from build123d import *

# Parameters (mm, degrees)
BOSS_EXTRU_1_DEPTH           = 20
ESQUISSE1_4_R                = 14
ENL_V_MAT_EXTRU_1_DEPTH      = 8
ESQUISSE3_R                  = 5
ENL_V_MAT_EXTRU_2_DEPTH      = 14
ENL_V_MAT_EXTRU_3_DEPTH      = 42.231056256
ENL_V_MAT_EXTRU_3_DEPTH_BACK = 42.231056256
ESQUISSE1_5_R                = 2
ESQUISSE1_6_R                = 4
ENL_V_MAT_EXTRU_4_DEPTH      = 2
ENL_V_START                  = 18
ESQUISSE1_7_R                = 4
ENL_V_MAT_EXTRU_5_DEPTH      = 2
ENL_V_MAT_EXTRU_6_REACH      = 43.231
ESQUISSE4_R                  = 10
ENL_V_MAT_EXTRU_7_DEPTH      = 8


with BuildPart() as part:
    # Esquisse1 → Boss.-Extru.1 (new body)
    with BuildSketch(Plane.XY):
        with BuildLine():
            Line((0, 20), (-30, 20))
            Line((-30, 20), (-30, -20))
            Line((-30, -20), (0, -20))
            ThreePointArc((0, -20), (20, 0), (0, 20))
        make_face()
    extrude(amount=BOSS_EXTRU_1_DEPTH)

    # Esquisse1<4> → Enlèv. mat.-Extru.1 (cut)
    with BuildSketch(Plane.XY):
        Circle(ESQUISSE1_4_R)
    extrude(amount=ENL_V_MAT_EXTRU_1_DEPTH, mode=Mode.SUBTRACT)

    # Esquisse3 → Enlèv. mat.-Extru.2 (cut)
    with BuildSketch(Plane.ZY.offset(30)):
        with Locations((10, 0)):
            Circle(ESQUISSE3_R)
    extrude(amount=-ENL_V_MAT_EXTRU_2_DEPTH, mode=Mode.SUBTRACT)

    # Esquisse1<5> → Enlèv. mat.-Extru.3 (cut, two sides: drawn at the far end of the back side and taken through both)
    with BuildSketch(Plane.XY.offset(-ENL_V_MAT_EXTRU_3_DEPTH_BACK)):
        with Locations((-23.5, 0)):
            Circle(ESQUISSE1_5_R)
    extrude(amount=ENL_V_MAT_EXTRU_3_DEPTH + ENL_V_MAT_EXTRU_3_DEPTH_BACK, mode=Mode.SUBTRACT)

    # Esquisse1<6> → Enlèv. mat.-Extru.4 (cut)
    with BuildSketch(Plane.XY):
        with Locations((-23.5, 0)):
            Circle(ESQUISSE1_6_R)
    extrude(amount=ENL_V_MAT_EXTRU_4_DEPTH, mode=Mode.SUBTRACT)

    # Esquisse1<7> → Enlèv. mat.-Extru.5 (cut)
    with BuildSketch(Plane.XY.offset(ENL_V_START)):
        with Locations((-23.5, 0)):
            Circle(ESQUISSE1_7_R)
    extrude(amount=ENL_V_MAT_EXTRU_5_DEPTH, mode=Mode.SUBTRACT)

    # Esquisse4 → Enlèv. mat.-Extru.6 (cut, up to next)
    with BuildSketch(Plane.XY.offset(20), mode=Mode.PRIVATE) as enl_v_mat_extru_6_sk1:
        Circle(ESQUISSE4_R)
    enl_v_mat_extru_6_tool1 = extrude(enl_v_mat_extru_6_sk1.sketch, amount=-ENL_V_MAT_EXTRU_6_REACH, mode=Mode.PRIVATE) & part.part
    add(enl_v_mat_extru_6_tool1.solids().sort_by_distance((0, 0, 20))[0], mode=Mode.SUBTRACT)

    # Esquisse5 → Enlèv. mat.-Extru.7 (cut)
    with BuildSketch(Plane.XY.offset(20)):
        with BuildLine():
            Line((0, 10), (0, 20))
            ThreePointArc((0, 20), (20, 0), (0, -20))
            Line((0, -20), (0, -10))
            ThreePointArc((0, -10), (-10, 0), (0, 10))
        make_face()
    extrude(amount=-ENL_V_MAT_EXTRU_7_DEPTH, mode=Mode.SUBTRACT)


solid = part.part
Check sheet for the modelled part. Datum: model origin and axes. Units: mm. A direction names the side the tool comes from. Give positions to 0.01 mm unless a question says otherwise; leave off trailing zeros. Write each loop counter-clockwise with the first axis right and the second up, starting at its lowest first coordinate (ties: lowest second). Pieces come first, ordered by that corner, then holes. Notation, with made-up numbers: (-3.5, 17) -> (5.5, 17) arc R20 ccw to (5.5, 53) -> close; hole circle Ø6 at (37, -11.75). An arc over 180 degrees is marked (long way). One line per item, written item: value. Start each with the question number.
Item 1: Section check B-B on x = -23.5. Record the cut outline in (y, z), then the cut area to 3 significant figures.
Item 2: Tool access check on faces 1 (the cylindrical face through (-23.098, -4.436, 12.307)), 2 (the cylindrical face through (-26.7, -2.4, 19)), 3 (the flat face through (0, 15, 16)), 4 (the cylindrical face through (12.932, -5.362, 3.944)). Record the directions out of +Z, -Z, +X, -X, +Y, -Y that give a thin tool (end or side, any length) a straight path to the whole face; none if there is none.
Item 3: Gauge pin test, flat ends, axial feed: pin 1 (9 mm diameter, centred on y = 13, z = 17.5, fed in from +X); pin 2 (9 mm diameter, centred on y = -16, z = 14, fed in from +X); pin 3 (18 mm diameter, centred on x = 0, y = 0, fed in from +Z); pin 4 (4 mm diameter, centred on x = -24, y = 1, fed in from -Z). Record the tip position at first contact, or that the pin passes through.
Item 4: Draft check along Y on faces 5 (the flat face through (-15, 0, 20)), 6 (the cylindrical face through (-21.592, 0.601, 3.685)), 7 (the flat face through (-15, 20, 10)). Enter one of: +Y half, -Y half, draft (parallel to the pull), parting line (faces both ways), or undercut.
Item 5: Section check A-A on z = 10. Record the cut outline in (x, y).
Item 6: Section check C-C on y = 0. State how many separate pieces and enclosed holes the cut face has, then the cut area to 3 significant figures.
Item 7: Material ranges on probe 1 along X at (y, z) = (0, 10.65); probe 2 along Y at (x, z) = (-23.5, 17.05); probe 3 along Y at (x, z) = (0, 10.5), recorded low to high. Write a range as from..to.
Item 8: Section check D-D on x = -17.5. Record the cut outline in (y, z), then the cut area to 3 significant figures.
Results list:
1. outline: (-20, 0) -> (-4, 0) -> (-4, 2) -> (-2, 2) -> (-2, 5.42) arc R5 cw to (-2, 14.58) -> (-2, 18) -> (-4, 18) -> (-4, 20) -> (-20, 20) -> close; (2, 2) -> (4, 2) -> (4, 0) -> (20, 0) -> (20, 20) -> (4, 20) -> (4, 18) -> (2, 18) -> (2, 14.58) arc R5 cw to (2, 5.42) -> close
1. area: 664 mm²
2. face 1: -X
2. face 2: +Z
2. face 3: +Z, +X, +Y, -Y
2. face 4: -Z
3. pin 1: x = 0
3. pin 2: x = 16.02
3. pin 3: through
3. pin 4: z = 2
4. face 5: draft
4. face 6: undercut
4. face 7: +Y half
5. outline: (-30, -20) -> (0, -20) arc R20 ccw to (0, 20) -> (-30, 20) -> (-30, 5) -> (-16, 5) -> (-16, -5) -> (-30, -5) -> close; hole circle Ø20 at (0, 0)
6. separate pieces: 4
6. enclosed holes: 0
6. area: 260 mm²
7. probe 1: -16..-10, 10..20
7. probe 2: -20..-2, 2..20
7. probe 3: -20..-10, 10..20
8. outline: (-20, 0) -> (20, 0) -> (20, 20) -> (-20, 20) -> close; hole circle Ø10 at (0, 10)
8. area: 721 mm²
